Answer from the drawing. Dimensions are ordinates in mm from the lowest x, y and z of the part. Round coordinates to 2 decimals unless told otherwise and drop trailing zeros. Order: outer loops, then holes, each group sorted by start corner. A loop starts at its lowest first (then second) coordinate and runs counter-clockwise, first axis right, second up.
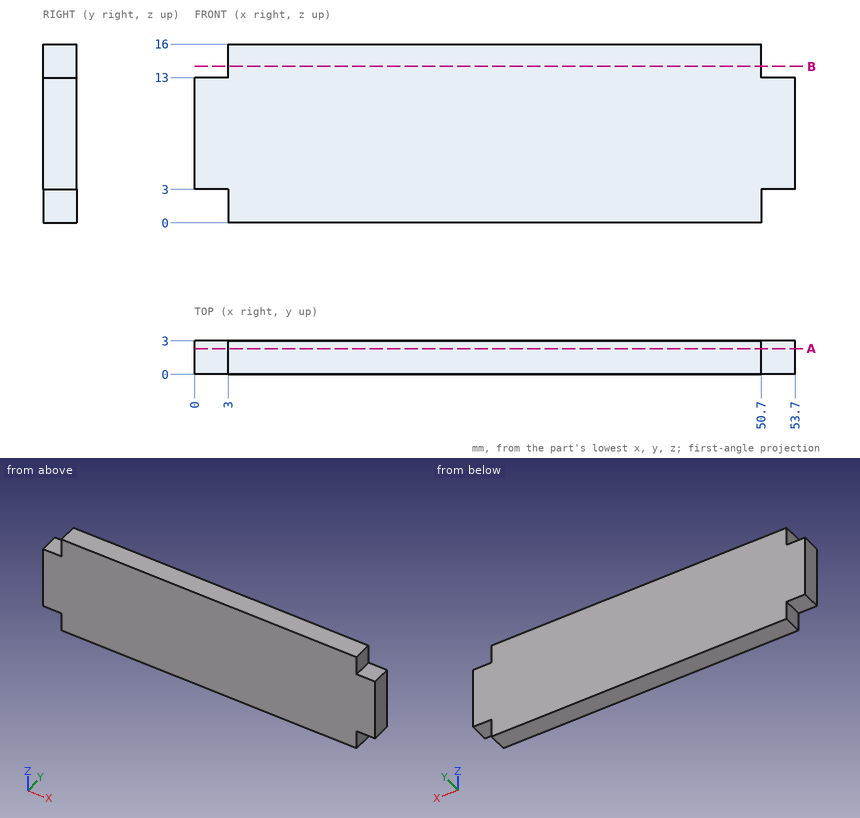
Q1. A cutting plane is placed at B-B, the plane z = 14. Give the vertices of the cut face in (x, y), plus the area to 3 significant figures.
Outcome:
outline: (3, 0) - (50.7, 0) - (50.7, 3) - (3, 3) - close
area: 143 mm2
Q2. A straight line is drawn through the part: probe 1 along X at (y, z) = (2.8, 1). Find the intervals that lie inside material, in ascending order.
Outcome:
probe 1: x = 3 to 50.7
Q3. Flat-ended cylindrical pins translate along their axes: pin 1 (1.5 mm diameter, centred on y = 2, z = 14, fed in from -X); pin 2 (0.9 mm diameter, centred on x = 1, y = 2, fed in from +Z); pin 3 (0.9 mm diameter, centred on x = 53, y = 1.5, fed in from -Z). Find the tip coordinate at first contact, or state that the pin passes through.
Outcome:
pin 1: stops at x = 3
pin 2: stops at z = 13
pin 3: stops at z = 3
Q4. A cutting plane is placed at A-A, the plane y = 2.3. Give the vertices of the cut face in (x, z).
Outcome:
outline: (0, 3) - (3, 3) - (3, 0) - (50.7, 0) - (50.7, 3) - (53.7, 3) - (53.7, 13) - (50.7, 13) - (50.7, 16) - (3, 16) - (3, 13) - (0, 13) - close
